Can you work these out from the drawing? Everything is in mm from the part's minimum corner. Give positions to 0.01 mm unless a question says otherwise; leave off trailing zeros. Write each loop counter-clockwise with the first axis right and the second up, starting at its lowest first coordinate (ties: lowest second). Pieces come first, ordered by that corner, then holes. Notation, with made-up numbers: (-12, 48.25) - (44, 48.25) arc R19 ccw to (44, 59.25) - close; hole circle Ø9 at (-28, 61). An arc over 180 degrees is marked (long way). Use a Markdown table: item, result.
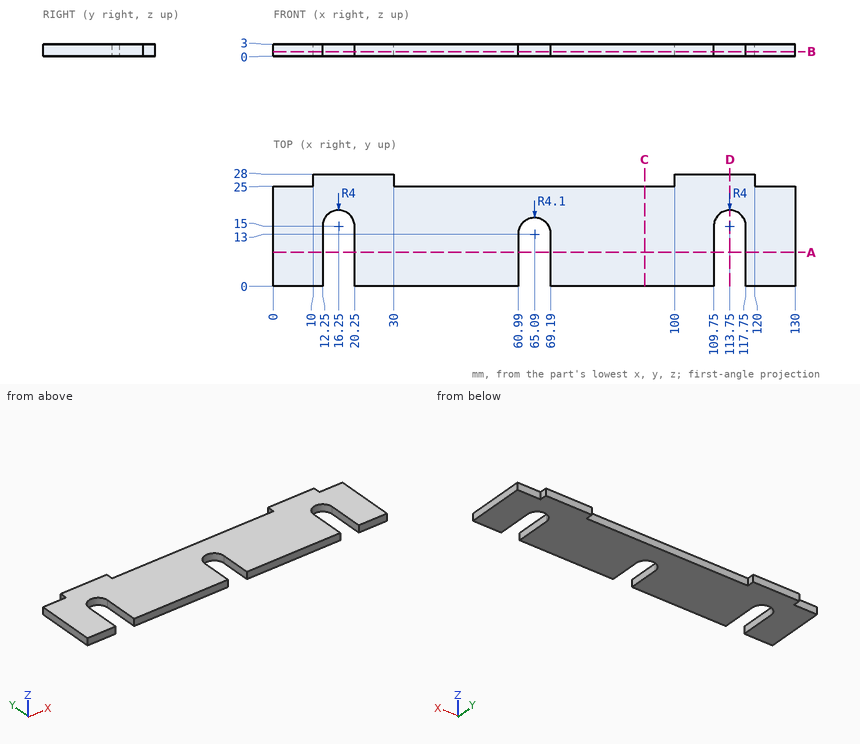
Item 1: If we section it at D-D, the plane x = 113.75: Write out the boundary of the cut face in (y, z).
Values:
| item | result |
|---|---|
| outline | (19, 0) - (28, 0) - (28, 3) - (19, 3) - close |
Item 2: I need wall thicknesses on line 1 along X through (y, z) = (2.5, 0.75); line 2 along X through (y, z) = (14.25, 2.25); line 3 along Y through (x, z) = (73.5, 0.7). Which ranges of each line are inside material? Lowest first, please. Write a range as [from, to].
Values:
| item | result |
|---|---|
| line 1 | x = [0, 12.25], [20.25, 60.99], [69.19, 109.75], [117.75, 130] |
| line 2 | x = [0, 12.25], [20.25, 61.19], [68.99, 109.75], [117.75, 130] |
| line 3 | y = [0, 25] |
Item 3: If we section it at C-C, the plane x = 92.5: Write out the boundary of the cut face in (y, z), plus the area to 3 significant figures.
Values:
| item | result |
|---|---|
| outline | (0, 0) - (25, 0) - (25, 3) - (0, 3) - close |
| area | 75.0 mm2 |
Item 4: If we section it at B-B, the plane z = 1.1: Write out the boundary of the cut face in (x, y), plus the area to 3 significant figures.
Values:
| item | result |
|---|---|
| outline | (0, 0) - (12.25, 0) - (12.25, 15) arc R4 cw to (20.25, 15) - (20.25, 0) - (60.99, 0) - (60.99, 13) arc R4.1 cw to (69.19, 13) - (69.19, 0) - (109.75, 0) - (109.75, 15) arc R4 cw to (117.75, 15) - (117.75, 0) - (130, 0) - (130, 25) - (120, 25) - (120, 28) - (100, 28) - (100, 25) - (30, 25) - (30, 28) - (10, 28) - (10, 25) - (0, 25) - close |
| area | 2,950 mm2 |
Item 5: If we section it at A-A, the plane y = 8.5: Write out the boundary of the cut face in (x, z), plus the area to 3 significant figures.
Values:
| item | result |
|---|---|
| outline | (0, 0) - (12.25, 0) - (12.25, 3) - (0, 3) - close; (20.25, 0) - (60.99, 0) - (60.99, 3) - (20.25, 3) - close; (69.19, 0) - (109.75, 0) - (109.75, 3) - (69.19, 3) - close; (117.75, 0) - (130, 0) - (130, 3) - (117.75, 3) - close |
| area | 317 mm2 |
Item 6: Will these pins go through, and if not, where does the flat tip stop? pin 1 Ø1.5 at (x, z) = (125, 2) entering from +Y; pin 2 Ø0.9 at (y, z) = (27, 1.5) entering from -X; pin 3 Ø1.5 at (y, z) = (26.5, 2) entering from +X.
Values:
| item | result |
|---|---|
| pin 1 | stops at y = 25 |
| pin 2 | stops at x = 10 |
| pin 3 | stops at x = 120 |
